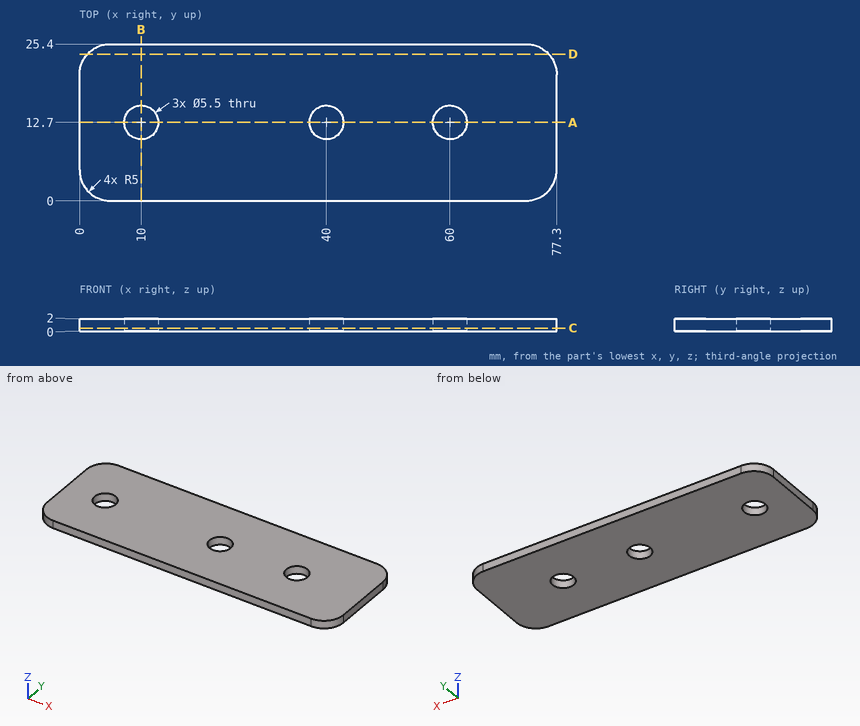
Part print with two shaded views. Sizes in mm from the minimum x, y, z corner. Coordinates: 2 decimals unless noted, no trailing zeros. Loops run counter-clockwise (first coordinate to the right, second up) from the corner with the lowest first, then second, coordinate; pieces in that order, holes last. Notation, with made-up numbers: (-21.5, -18) -> (8.5, -18) arc R21 ccw to (8.5, 9) -> close; hole circle Ø3 at (-38.5, 89). An arc over 180 degrees is marked (long way). Answer as a JSON object with one key per item and string values.
Q1. Cut at B-B (x = 10). List the corners of the cut face in (y, z).
Report:
{"outline": "(0, 0) -> (9.95, 0) -> (9.95, 2) -> (0, 2) -> close; (15.45, 0) -> (25.4, 0) -> (25.4, 2) -> (15.45, 2) -> close"}
Q2. Cut at A-A (y = 12.7). List the corners of the cut face in (x, z), and give its area (3 significant figures).
Report:
{"outline": "(0, 0) -> (7.25, 0) -> (7.25, 2) -> (0, 2) -> close; (12.75, 0) -> (37.25, 0) -> (37.25, 2) -> (12.75, 2) -> close; (42.75, 0) -> (57.25, 0) -> (57.25, 2) -> (42.75, 2) -> close; (62.75, 0) -> (77.3, 0) -> (77.3, 2) -> (62.75, 2) -> close", "area": "122 mm2"}
Q3. Cut at D-D (y = 23.75). List the corners of the cut face in (x, z), and give its area (3 significant figures).
Report:
{"outline": "(1.29, 0) -> (76.01, 0) -> (76.01, 2) -> (1.29, 2) -> close", "area": "149 mm2"}
Q4. Cut at C-C (z = 0.5). List the corners of the cut face in (x, y), and give its area (3 significant figures).
Report:
{"outline": "(0, 5) arc R5 ccw to (5, 0) -> (72.3, 0) arc R5 ccw to (77.3, 5) -> (77.3, 20.4) arc R5 ccw to (72.3, 25.4) -> (5, 25.4) arc R5 ccw to (0, 20.4) -> close; hole circle Ø5.5 at (10, 12.7); hole circle Ø5.5 at (40, 12.7); hole circle Ø5.5 at (60, 12.7)", "area": "1,870 mm2"}
Q5. Probe probe 1 along Y at (x, z) = (10, 1.05); probe 2 along X at (y, z) = (13.5, 1.75); probe 3 along X at (y, z) = (23, 1.5). List the from-to ranges inside material, lowest first.
Report:
{"probe 1": "y = 0 to 9.95, 15.45 to 25.4", "probe 2": "x = 0 to 7.37, 12.63 to 37.37, 42.63 to 57.37, 62.63 to 77.3", "probe 3": "x = 0.73 to 76.57"}
